Autodesk Fusion 360 part; units mm, degrees
ref_plane "WorkPlane1" through (0, 60, 0) normal (0, 1, 0) x (0, 0, 1)
sketch "Sketch1" plane through (0, 60, 0) normal (0, 1, 0) x (1, 0, 0)
  line L0 (20, 28.7228) -> (20, -28.7228)
  line L1 (25, 24.4949) -> (25, -24.4949)
  arc A0 (25, 24.4949) -> (25, -24.4949) centre (0, 0) ccw
  arc A1 (25, 16.5831) -> (25, -16.5831) centre (0, 0) ccw
  dimension "d2" = 60
  dimension "d3" = 70
  dimension "d4" = 20
  dimension "d5" = 5
extrude "Extrude1" add sketch "Sketch1" along normal blind 100 contours L0 L1 A0 A1 | L0 A0 A1 | L0 L1 A1 | L0 L1 A0 A1
extrude "Extrude2" add sketch "Sketch1" against normal blind 60 contours L0 L1 A0 A1 | L0 L1 A1 | L0 L1 A0 A1
ref_plane "WorkPlane2" through (0, 124.607, 35) normal (0, 0, 1) x (-1, 0, 0)
sketch "Sketch2" plane through (0, 124.607, 35) normal (0, 0, 1) x (1, 0, 0)
  line L0 (20, -64.607) -> (-35, -64.607)
  line L1 (20, -64.607) -> (20, -124.607)
  line L2 (20, -124.607) -> (25, -124.607)
  line L3 (25, -124.607) -> (25, 35.393)
  line L4 (25, 35.393) -> (-35, 35.393)
  line L5 (25, 35.393) -> (25, -124.607)
  line L6 (20, -124.607) -> (25, -124.607)
  line L7 (20, -124.607) -> (20, -64.607)
  line L8 (-10, -9.607) -> (10, -9.607)
  line L9 (10, -9.607) -> (10, -19.607)
  line L10 (10, -19.607) -> (-10, -19.607)
  line L11 (-10, -19.607) -> (-10, -9.607)
  dimension "d11" = 45
  dimension "d12" = 10
  dimension "d13" = 20
  dimension "d14" = 15
ref_plane "WorkPlane3" through (0, 127.6389, 35) normal (0, 0, 1) x (-1, 0, 0)
sketch "Sketch6" plane through (0, 127.6389, 35) normal (0, 0, 1) x (1, 0, 0)
  line L0 (20, -127.6389) -> (25, -127.6389)
  line L1 (20, -67.6389) -> (20, -127.6389)
  line L2 (25, 32.3611) -> (25, -127.6389)
  line L3 (20, -67.6389) -> (-35, -67.6389)
  line L4 (25, 32.3611) -> (-35, 32.3611)
  line L5 (-35, -67.6389) -> (-35, 32.3611)
  line L6 (25, 32.3611) -> (20, 32.3611)
  line L7 (20, 32.3611) -> (20, -127.6389)
  line L8 (20, -127.6389) -> (25, -127.6389)
  line L9 (25, -127.6389) -> (25, 32.3611)
extrude "Extrude9" add sketch "Sketch6" against normal blind 15 contours L0 L1 L2 L4 L6 L7 L8 L9
extrude "Extrude10" add sketch "Sketch6" along normal blind 5 contours L0 L1 L2 L4 L6 L7 L8 L9
mirror "Mirror2" about plane through (0, 0, 0) normal (0, 0, 1) of bodies 1 merged
sketch "Sketch7" plane through (25, 0, 0) normal (1, 0, 0) x (0, 0, -1)
  line L0 (40, 160) -> (-40, 160)
  line L1 (-40, 160) -> (-40, 0)
  line L2 (-40, 0) -> (40, 0)
  line L3 (40, 0) -> (40, 160)
  line L4 (-30, 40) -> (30, 40)
  line L5 (30, 40) -> (30, 30)
  line L6 (30, 30) -> (-30, 30)
  line L7 (-30, 30) -> (-30, 40)
  line L8 (28.7228, 160) -> (28.7228, 60)
  line L9 (35, 60) -> (-35, 60)
  line L10 (-28.7228, 60) -> (-28.7228, 160)
  line L11 (35, 160) -> (-35, 160)
  dimension "d41" = 60
  dimension "d42" = 10
  dimension "d43" = 10
  dimension "d45" = 20
extrude "Extrude11" cut sketch "Sketch7" against normal through all contours L4 L5 L6 L7
sketch "Sketch8" plane through (20, 0, 0) normal (-1, 0, 0) x (0, 0, 1)
  line L0 (30, 40) -> (30, 30)
  line L1 (30, 30) -> (-30, 30)
  line L2 (-30, 30) -> (-30, 40)
  line L3 (-30, 40) -> (30, 40)
  line L4 (-40, 0) -> (40, 0)
  line L5 (40, 0) -> (40, 160)
  line L6 (40, 160) -> (28.7228, 160)
  line L7 (28.7228, 160) -> (28.7228, 60)
  line L8 (28.7228, 60) -> (22.3607, 60)
  line L9 (22.3607, 60) -> (22.3607, 160)
  line L10 (22.3607, 160) -> (-22.3607, 160)
  line L11 (-22.3607, 160) -> (-22.3607, 60)
  line L12 (-22.3607, 60) -> (-28.7228, 60)
  line L13 (-28.7228, 60) -> (-28.7228, 160)
  line L14 (-28.7228, 160) -> (-40, 160)
  line L15 (-40, 160) -> (-40, 0)
  line L16 (-40, 5) -> (40, 5)
  line L17 (40, 5) -> (40, 0)
  line L18 (40, 0) -> (-40, 0)
  line L19 (-40, 0) -> (-40, 5)
  dimension "d47" = 5
extrude "Extrude12" add sketch "Sketch8" along normal blind 55 contours L4 L5 L15 L16 L17 L18 L19
sketch "Sketch9" plane through (0, 5, 0) normal (0, 1, 0) x (-1, 0, 0)
  line L0 (-20, 40) -> (-20, -40)
  line L1 (-20, -40) -> (35, -40)
  line L2 (35, -40) -> (35, 40)
  line L3 (35, 40) -> (-20, 40)
  circle A0 centre (-15, 35) radius 3.225
  circle A1 centre (30, 35) radius 3.225
  circle A2 centre (30, -35) radius 3.225
  circle A3 centre (-15, -35) radius 3.225
  dimension "d50" = 6.45
  dimension "d51" = 5
  dimension "d52" = 5
  dimension "d53" = 6.45
  dimension "d54" = 5
  dimension "d57" = 6.45
  dimension "d58" = 6.45
  dimension "d59" = 5
  dimension "d60" = 5
  dimension "d61" = 5
  dimension "d62" = 5
extrude "Extrude13" cut sketch "Sketch9" against normal blind 5 contours A0 | A1 | A2 | A3
Geometry: final body of the model. Coordinates: model frame, mm. A direction names the side the tool comes from. Give positions to 0.01 mm unless a question says otherwise; leave off trailing zeros. Loops run counter-clockwise (first coordinate to the right, second up) from the corner with the lowest first, then second, coordinate; pieces in that order, holes last. Notation, with made-up numbers: (-32.75, 18.25) -> (-1.75, 18.25) arc R13 ccw to (-1.75, 23.25) -> close; hole circle Ø5 at (27, 77). An arc over 180 degrees is marked (long way). Return JSON: item names as keys, results as strings.
Item 1: Section C-C, the plane x = 5. Output: boundary loops of the cut face in (y, z), plus the area to 3 significant figures.
Filled in:
{"outline": "(0, -40) -> (5, -40) -> (5, 40) -> (0, 40) -> close; (60, -34.64) -> (160, -34.64) -> (160, -29.58) -> (60, -29.58) -> close; (60, 29.58) -> (160, 29.58) -> (160, 34.64) -> (60, 34.64) -> close", "area": "1,410 mm^2"}
Item 2: Access query for faces 4 (the flat face through (22, 57, -40)), 5 (the flat face through (22, 56, 40)), 6 (the cylindrical face through (-29.984, 109.3, 0.966)), 7 (the flat face through (-30.04, 60, -2.76)), 8 (the flat face through (23, 30, 0)). Directions: +Z, -Z, +X, -X, +Y, -Y. A direction counts if a zero-diameter tool reaches every point of the face in a straight line with its end or side. Return the directions, or none.
Filled in:
{"face 4": "-Z, +X, -X, +Y, -Y", "face 5": "+Z, +X, -X, +Y, -Y", "face 6": "+Y", "face 7": "+Z, -Z, -X", "face 8": "+X, -X"}
Item 3: Mould query, pull axis Y, two halves, no side actions, for faces 1 (the flat face through (23, 35, 30)), 2 (the cylindrical face through (-29.6, 2.5, -31.8)), 3 (the flat face through (22, 160, 0)). Classes: released by +Y, released by -Y, zero draft, split by the parting line, or undercut.
Filled in:
{"face 1": "undercut", "face 2": "zero draft", "face 3": "released by +Y"}
Item 4: Pin query (flat end, axial travel): P1, Ø24, axis at y = 45.5, z = 2.5, coming from the -X side; P2, Ø6, axis at x = 15, z = 35, coming from the -Y side; P3, Ø3, axis at x = 12.5, z = 17.5, coming from the +Y side. Return the tip coordinate at first contact, or that it passes through.
Filled in:
{"P1": "x = 20", "P2": "through", "P3": "y = 5"}
Item 5: Line query: line 1 (Z direction, x = -30, y = 1.55) (3 decimals); line 2 (Y direction, x = 21, z = -2.5); line 3 (Y direction, x = -22, z = -25). Output: solid intervals per line, ascending.
Filled in:
{"line 1": "-40 to -38.225, -31.775 to 31.775, 38.225 to 40", "line 2": "0 to 30, 40 to 160", "line 3": "0 to 5, 60 to 160"}
Item 6: Section A-A, the plane z = 0. Output: boundary loops of the cut face in (x, y), plus the area to 4 significant figures.
Filled in:
{"outline": "(-35, 0) -> (25, 0) -> (25, 30) -> (20, 30) -> (20, 5) -> (-35, 5) -> close; (-35, 60) -> (-30, 60) -> (-30, 160) -> (-35, 160) -> close; (20, 40) -> (25, 40) -> (25, 160) -> (20, 160) -> close", "area": "1,525 mm^2"}
Item 7: Section B-B, the plane x = 15. Output: boundary loops of the cut face in (y, z) (3 decimals).
Filled in:
{"outline": "(0, -40) -> (5, -40) -> (5, -38.225) -> (0, -38.225) -> close; (0, -31.775) -> (5, -31.775) -> (5, 31.775) -> (0, 31.775) -> close; (0, 38.225) -> (5, 38.225) -> (5, 40) -> (0, 40) -> close; (60, -31.623) -> (160, -31.623) -> (160, -25.981) -> (60, -25.981) -> close; (60, 25.981) -> (160, 25.981) -> (160, 31.623) -> (60, 31.623) -> close"}
Item 8: Section D-D, the plane y = 102. Output: boundary loops of the cut face in (x, z), plus the area to 3 significant figures.
Filled in:
{"outline": "(20, -40) -> (25, -40) -> (25, 40) -> (20, 40) -> (20, 28.72) arc R35 ccw (long way) to (20, -28.72) -> close; hole (20, -22.36) -> (20, 22.36) arc R30 ccw (long way) to start", "area": "1,130 mm^2"}
